Model file for the job. Use its own axes, mm. A direction names the side the tool comes from. Coordinates: 2 decimals unless noted, no trailing zeros. Order: outer loops, then holes, each group sorted by start corner. A loop starts at its lowest first (then second) coordinate and runs counter-clockwise, first axis right, second up. Notation, with made-up numbers: M 83,-1 L 127,-1 A29 cw 127,25 Z; hole C 6.5,-15.75 d11. An arc over 180 degrees is marked long. Return JSON: item names as keys, results as strings.
```python
from build123d import *

# Parameters (mm, degrees)
BOSS_EXTRUDE1_START = -4
SKETCH1_W           = 12
SKETCH1_H           = 12
BOSS_EXTRUDE1_DEPTH = 16.6
SKETCH2_W           = 5.4
SKETCH2_H           = 5.4
CUT_EXTRUDE1_DEPTH  = 12
BOSS_EXTRUDE2_START = 9.6
BOSS_EXTRUDE2_DEPTH = 3
SKETCH4_R           = 1.8
CUT_EXTRUDE2_DEPTH  = 25.2


with BuildPart() as part:
    # Sketch1 → Boss-Extrude1 (new body)
    with BuildSketch(Plane.XY.offset(BOSS_EXTRUDE1_START)):
        Rectangle(SKETCH1_W, SKETCH1_H)
    extrude(amount=BOSS_EXTRUDE1_DEPTH)

    # Sketch2 → Cut-Extrude1 (cut, symmetric)
    with BuildSketch(Plane(origin=(0, 0, 0), x_dir=(1, 0, 0), z_dir=(0, 1, 0))):
        Rectangle(SKETCH2_W, SKETCH2_H)
    extrude(amount=CUT_EXTRUDE1_DEPTH, both=True, mode=Mode.SUBTRACT)

    # Sketch3 → Boss-Extrude2 (add)
    with BuildSketch(Plane.XY.offset(BOSS_EXTRUDE2_START)):
        Polygon((-5, 6), (5, 6), (0, 65), (-16, 65), align=None)
    extrude(amount=BOSS_EXTRUDE2_DEPTH)

    # Sketch4 → Cut-Extrude2 (cut, symmetric)
    with BuildSketch(Plane.XY):
        with Locations((-8.5, 60)):
            Circle(SKETCH4_R)
    extrude(amount=CUT_EXTRUDE2_DEPTH, both=True, mode=Mode.SUBTRACT)


solid = part.part
```
Item 1: Saw through at C-C (x = 4.25). Write the cut outline in (y, z), and give its area (3 significant figures).
Check result:
{"outline": "M -6,-4 L 6,-4 L 6,9.6 L 14.85,9.6 L 14.85,12.6 L -6,12.6 Z", "area": "226 mm2"}
Item 2: Saw through at B-B (y = 60). Write the cut outline in (x, z), and give its area (3 significant figures).
Check result:
{"outline": "M -15.07,9.6 L -10.3,9.6 L -10.3,12.6 L -15.07,12.6 Z; M -6.7,9.6 L 0.42,9.6 L 0.42,12.6 L -6.7,12.6 Z", "area": "35.7 mm2"}
Item 3: Saw through at A-A (x = -8.5). Write the cut outline in (y, z).
Check result:
{"outline": "M 24.77,9.6 L 58.2,9.6 L 58.2,12.6 L 24.77,12.6 Z; M 61.8,9.6 L 65,9.6 L 65,12.6 L 61.8,12.6 Z"}
Item 4: Wall check: line 1 (X direction, y = 2.5, z = -2); line 2 (Z direction, x = -1.25, y = 1.5); line 3 (Y direction, x = 1, z = 4.5). Give the ranges that are in metal, low to high.
Check result:
{"line 1": "x = -6 to -2.7, 2.7 to 6", "line 2": "z = -4 to -2.7, 2.7 to 12.6", "line 3": "y = -6 to 6"}
Item 5: 3-axis set-ups, long thin cutter, end or side, ignore diameter. For faces 5 (the flat face through (2.535, 35.087, 11.079)), 6 (the flat face through (2.7, 0, 0)), 7 (the flat face through (-6, 0, 4)): which of +Z, -Z, +X, -X, +Y, -Y reach the whole face in a straight line?
Check result:
{"face 5": "+Z, -Z, +X, +Y", "face 6": "+Y, -Y", "face 7": "+Z, -Z, -X, -Y"}
Item 6: Drop flat-ended pins along their axis: pin 1 Ø6 at (y, z) = (0, 2.5) entering from -X; pin 2 Ø9.5 at (x, z) = (2.5, 0.5) entering from +Y; pin 3 Ø8 at (x, y) = (-13, 35.5) entering from -Z. Give the stop position or say it passes through.
Check result:
{"pin 1": "stops at x = -6", "pin 2": "stops at y = 6", "pin 3": "stops at z = 9.6"}
Item 7: Pull direction X, two halves, no side cores. Call faces 1 (the flat face through (6, 0, 4)), 2 (the flat face through (-2.7, 0, 0)), 3 (the flat face through (0, 0, 2.7)), 4 (the flat face through (-6, 36, 9.6)): +X half, -X half, draft (parallel to the pull), parting line (faces both ways), or undercut.
Check result:
{"face 1": "+X half", "face 2": "undercut", "face 3": "undercut", "face 4": "draft"}
Item 8: Saw through at D-D (z = 3.5). Write the cut outline in (x, y).
Check result:
{"outline": "M -6,-6 L 6,-6 L 6,6 L -6,6 Z"}
